Design review of the part built by this model. Coordinates are the model's own, in mm. Face numbers are marked on the shaded views. A direction names the side the tool comes from. Round coordinates to 2 decimals unless told otherwise and drop trailing zeros. Loops run counter-clockwise (first coordinate to the right, second up) from the corner with the lowest first, then second, coordinate; pieces in that order, holes last. Notation, with made-up numbers: (86, 62) -> (117, 62) arc R16 cw to (117, 87) -> close; hole circle Ø1 at (-10.75, 39). An arc over 180 degrees is marked (long way). Answer as CSV lines item,"result". Start each with the question number.
```python
from build123d import *

# Parameters (mm, degrees)
F1_DEPTH    = 116.84
F2_W        = 86.36
F2_H        = 15.24
F3_DEPTH    = 2.54
F4_W        = 86.36
F4_H        = 15.24
F5_DEPTH    = 2.54
F6_T1_DEPTH = 148.0482991577
F6_T3_DEPTH = 112.4882991577
F7_SIZE     = 5.08


# Not quite as in the source:
# - a fillet or chamfer that OpenCascade refuses, or shapes differently, is made with other operations: its cross-section is extruded or revolved along the edge and cut away or added


with BuildPart() as f1:
    # F0 (on Front) → F1 (new body)
    with BuildSketch(Plane.XZ):
        Polygon((43.18, 0), (36.83, 0), (29.21, -13.1982271537), (13.97, -13.1982271537), (6.35, 0), (0, 0), (-6.35, 0), (-13.97, -13.1982271537), (-29.21, -13.1982271537), (-36.83, 0), (-43.18, 0), (-43.18, -15.24), (0, -15.24), (43.18, -15.24), align=None)
    extrude(amount=F1_DEPTH)

    # F2 (on face) → F3 (join)
    with BuildSketch(Plane.XZ.offset(116.84)):
        with Locations((0, -7.62)):
            Rectangle(F2_W, F2_H)
    extrude(amount=F3_DEPTH)

    # F4 (on face) → F5 (join)
    with BuildSketch(Plane(origin=(0, 0, 0), x_dir=(-1, 0, 0), z_dir=(0, 1, 0))):
        with Locations((0, -7.62)):
            Rectangle(F4_W, F4_H)
    extrude(amount=F5_DEPTH)

    # F6: chamfer of 5.08 on 4 edges, made by hand

    # F6_s2 → F6_t1 (cut)
    with BuildSketch(Plane.XZ.offset(-15.6041495789)):
        Polygon((-38.1, 0), (-43.18, -5.08), (-43.18, 0), align=None)
        Polygon((38.1, 0), (43.18, -5.08), (43.18, 0), align=None)
    extrude(amount=F6_T1_DEPTH, mode=Mode.SUBTRACT)

    # F6_s4 → F6_t3 (cut)
    with BuildSketch(Plane.YZ.offset(-56.2441495789)):
        Polygon((-114.3, 0), (-119.38, -5.08), (-119.38, 0), align=None)
        Polygon((-2.54, 0), (2.54, -5.08), (2.54, 0), align=None)
    extrude(amount=F6_T3_DEPTH, mode=Mode.SUBTRACT)

    # F7
    f7_edges = [f1.edges().sort_by_distance(p)[0] for p in [
        (-43.18, -119.38, -10.16),
        (43.18, -119.38, -10.16),
        (43.18, 2.54, -10.16),
        (-43.18, 2.54, -10.16),
    ]]
    chamfer(f7_edges, length=F7_SIZE)


solid = f1.part
```
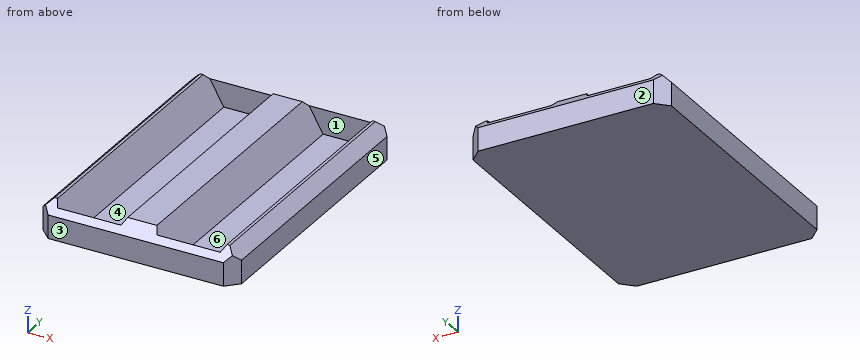
Q1. Add section A-A, the plane x = -17.5. Give the boundary of the cut face in (y, z), and give its area (3 significant figures).
Q2. Mouldability with a two-part tool opening along Y and no side actions: class the marked faces 1, 2, 3 and 4 as pulls with the +Y half, pulls with the -Y half, needs draft (parallel to the pull), parting line crosses it, or undercut.
Q3. For pin 1 Ø10 at (x, y) = (18.5, -37) entering from +Z; pin 2 Ø1 at (x, z) = (-1.5, -2) entering from -Y; pin 3 Ø12 at (x, y) = (-23.5, -37.5) entering from +Z; pin 4 Ø3 at (x, z) = (-28, -5) entering from +Y, all flat-tipped, find the tip position at first contact; note any pin that passes through.
Q4. Machinability: for the marked faces 5 and 6, which of the approach directions +Z, -Z, +X, -X, +Y, -Y give a long, thin tool a straight path to every point of the face, cutting with its end or side? Answer none if there is none.
Q5. Add section B-B, the plane y = -55.5. Give the boundary of the cut face in (x, z), and give its area (3 significant figures).
Q6. Add section C-C, the plane z = -9.75. Give the boundary of the cut face in (x, y), and give its area (3 significant figures).
Q7. To check wall thickness, follow probe 1 along Y at (x, z) = (-19.5, -8); probe 2 along X at (y, z) = (-30.5, -6.5); probe 3 along X at (y, z) = (-72, -9). State the ranges of each line that lie inside material, in increasing order. Write a range as from..to.
Worked answers:
1,outline,"(-119.38, -15.24) -> (2.54, -15.24) -> (2.54, -5.08) -> (0, -2.54) -> (0, -13.2) -> (-116.84, -13.2) -> (-116.84, -2.54) -> (-119.38, -5.08) -> close"
1,area,"297 mm^2"
2,face 1,"undercut"
2,face 2,"pulls with the +Y half"
2,face 3,"pulls with the -Y half"
2,face 4,"undercut"
3,pin 1,"stops at z = -12.38"
3,pin 2,"stops at y = -116.8"
3,pin 3,"stops at z = -12.7"
3,pin 4,"stops at y = 2.54"
4,face 5,"+Z, -Z, +X, +Y, -Y"
4,face 6,"+Z"
5,outline,"(-43.18, -15.24) -> (43.18, -15.24) -> (43.18, -5.08) -> (38.1, 0) -> (36.83, 0) -> (29.21, -13.2) -> (13.97, -13.2) -> (6.35, 0) -> (-6.35, 0) -> (-13.97, -13.2) -> (-29.21, -13.2) -> (-36.83, 0) -> (-38.1, 0) -> (-43.18, -5.08) -> close"
5,area,"687 mm^2"
6,outline,"(-43.18, -114.3) -> (-38.1, -119.38) -> (38.1, -119.38) -> (43.18, -114.3) -> (43.18, -2.54) -> (38.1, 2.54) -> (-38.1, 2.54) -> (-43.18, -2.54) -> close; hole (-31.2, -116.84) -> (-11.98, -116.84) -> (-11.98, 0) -> (-31.2, 0) -> close; hole (11.98, -116.84) -> (31.2, -116.84) -> (31.2, 0) -> (11.98, 0) -> close"
6,area,"5,990 mm^2"
7,probe 1,"y = -119.38..-116.84, 0..2.54"
7,probe 2,"x = -43.18..-33.08, -10.1..10.1, 33.08..43.18"
7,probe 3,"x = -43.18..-31.63, -11.55..11.55, 31.63..43.18"
